Geometry: final body of the model. Coordinates: model frame, mm. Face numbers are marked on the shaded views. A direction names the side the tool comes from. Round coordinates to 2 decimals unless told otherwise and drop trailing zeros. Loops run counter-clockwise (first coordinate to the right, second up) from the corner with the lowest first, then second, coordinate; pieces in that order, holes last. Notation, with made-up numbers: (65.25, 33) - (84.25, 33) arc R37 cw to (84.25, 70) - close; hole circle Ø2 at (-24.5, -13.75). An arc over 180 degrees is marked (long way). Answer in a Markdown table with one row per item. Add a question column.
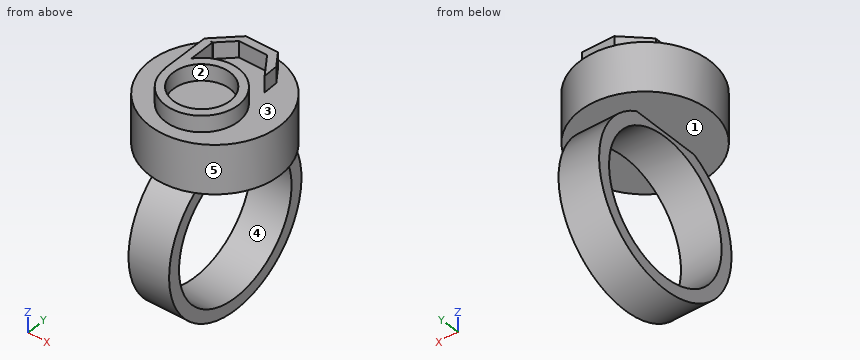
from build123d import *

# Parameters (mm, degrees)
F0_R      = 12.7
F1_DEPTH  = 6.35
F2_R      = 10.795
F3_DEPTH  = 55.83853
F6_R      = 10.156235
F7_DEPTH  = 7.62
F9_R      = 5.715
F10_DEPTH = 2.54
F11_R     = 4.445
F12_DEPTH = 25.4
F13_W     = 1.27
F13_H     = 7.62
F14_DEPTH = 2.54
F16_DEPTH = 2.54
F17_W     = 5.072208
F17_H     = 1.261867
F18_DEPTH = 2.54
F20_DEPTH = 2.54


with BuildPart() as f1:
    # F0 (on Right) → F1 (new body)
    with BuildSketch(Plane.YZ):
        Circle(F0_R)
    extrude(amount=F1_DEPTH)

    # F2 (on Right) → F3 (cut)
    with BuildSketch(Plane.YZ):
        Circle(F2_R)
    extrude(amount=F3_DEPTH, mode=Mode.SUBTRACT)

    # F6 (on offset) → F7 (join)
    with BuildSketch(Plane.XY.offset(11.43)):
        with Locations((3.156903, 0)):
            Circle(F6_R)
    extrude(amount=F7_DEPTH)

    # F9 (on offset) → F10 (join)
    with BuildSketch(Plane.XY.offset(19.05)):
        with Locations((3.159848, -2.503511)):
            Circle(F9_R)
    extrude(amount=F10_DEPTH)

    # F11 (on offset) → F12 (cut)
    with BuildSketch(Plane.XY.offset(19.05)):
        with Locations((3.132005, -2.497431)):
            Circle(F11_R)
    extrude(amount=F12_DEPTH, mode=Mode.SUBTRACT)

    # F13 (on offset) → F14 (join)
    with BuildSketch(Plane.XY.offset(19.05)):
        with Locations((-1.985011, 1.270657)):
            Rectangle(F13_W, F13_H)
    extrude(amount=F14_DEPTH)

    # F15 (on offset) → F16 (join)
    with BuildSketch(Plane.XY.offset(19.05)):
        Polygon((0.990725, 8.591608), (-2.646419, 5.053434), (-1.335068, 5.102919), (2.251208, 8.591608), align=None)
    extrude(amount=F16_DEPTH)

    # F17 (on offset) → F18 (join)
    with BuildSketch(Plane.XY.offset(19.05)):
        with Locations((3.487949, 7.974144)):
            Rectangle(F17_W, F17_H)
    extrude(amount=F18_DEPTH)

    # F19 (on offset) → F20 (join)
    with BuildSketch(Plane.XY.offset(19.05)):
        Polygon((6.024053, 8.580334), (5.277778, 7.432801), (7.72065, 3.951121), (7.633835, 6.286007), align=None)
    extrude(amount=F20_DEPTH)


solid = f1.part
1) Contact query for flat-ended pins moving along their axis: pin 1 Ø12 at (y, z) = (5.5, -8.5) entering from -X; pin 2 Ø3 at (y, z) = (-0.5, 21) entering from -X; pin 3 Ø2 at (y, z) = (-4.5, 15.5) entering from +X; pin 4 Ø8 at (y, z) = (-0.5, -6) entering from -X. Output: stop coordinate, or through.
2) Pull-direction query (X, two-part tool) for the marked faces 3, 4 and 5; classes: pulls with the +X half, pulls with the -X half, needs draft (parallel to the pull), parting line crosses it, or undercut.
3) Section D-D, the plane y = 0. Return the cut outline in (x, z) (3 decimals).
4) Section C-C, the plane x = 4.25. Return the cut outline in (y, z) (3 decimals).
5) Material intervals for line 1 along Y through (x, z) = (2.5, 0) (3 decimals); line 2 along Z through (x, y) = (7.75, -6); line 3 along Y through (x, z) = (0.75, 5), sorted ascending. Write a range as from..to.
6) Reachability of the marked faces 1 and 2 from +Z, -Z, +X, -X, +Y, -Y: full face, straight path, thin tool, end or side. Return the list, or none.
7) Section B-B, the plane z = 0. Return the cut outline in (x, y) (3 decimals), and give its area (3 significant figures).
8) Section A-A, the plane y = 2.75. Return the cut outline in (x, z).
Evaluation:
| question | item | result |
|---|---|---|
| 1 | pin 1 | stops at x = 0 |
| 1 | pin 2 | stops at x = -2.62 |
| 1 | pin 3 | stops at x = 12.69 |
| 1 | pin 4 | passes through |
| 2 | face 3 | undercut |
| 2 | face 4 | needs draft |
| 2 | face 5 | parting line crosses it |
| 3 | outline | (-6.999, 11.43) - (0, 11.43) - (0, 10.795) - (6.35, 10.795) - (6.35, 11.43) - (13.313, 11.43) - (13.313, 19.05) - (8.297, 19.05) - (8.297, 21.59) - (6.809, 21.59) - (6.809, 19.05) - (-0.545, 19.05) - (-0.545, 21.59) - (-2.62, 21.59) - (-2.62, 19.05) - (-6.999, 19.05) - close; (0, -12.7) - (6.35, -12.7) - (6.35, -10.795) - (0, -10.795) - close |
| 4 | outline | (-10.097, 11.43) - (-5.536, 11.43) arc R12.7 ccw (long way) to (5.536, 11.43) - (10.097, 11.43) - (10.097, 19.05) - (8.605, 19.05) - (8.605, 21.59) - (7.343, 21.59) - (7.343, 19.05) - (3.107, 19.05) - (3.107, 21.59) - (1.805, 21.59) - (1.805, 19.05) - (-6.8, 19.05) - (-6.8, 21.59) - (-8.114, 21.59) - (-8.114, 19.05) - (-10.097, 19.05) - close; hole circle Ø21.59 at (0, 0) |
| 5 | line 1 | y = -12.7..-10.795, 10.795..12.7 |
| 5 | line 2 | z = 11.43..19.05 |
| 5 | line 3 | y = -11.67..-9.57, 9.57..11.67 |
| 6 | face 1 | none |
| 6 | face 2 | +Z |
| 7 | outline | (0, -12.7) - (6.35, -12.7) - (6.35, -10.795) - (0, -10.795) - close; (0, 10.795) - (6.35, 10.795) - (6.35, 12.7) - (0, 12.7) - close |
| 7 | area | 24.2 mm² |
| 8 | outline | (-6.62, 11.43) - (0, 11.43) - (0, 10.44) - (6.35, 10.44) - (6.35, 11.43) - (12.93, 11.43) - (12.93, 19.05) - (5.41, 19.05) - (5.41, 21.59) - (0.91, 21.59) - (0.91, 19.05) - (-1.35, 19.05) - (-1.35, 21.59) - (-2.62, 21.59) - (-2.62, 19.05) - (-6.62, 19.05) - close; (0, -12.4) - (6.35, -12.4) - (6.35, -10.44) - (0, -10.44) - close |
